Part model, mm, in its own coordinate system. A direction names the side the tool comes from. Give positions to 0.01 mm unless a question says otherwise; leave off trailing zeros. Write each loop counter-clockwise with the first axis right and the second up, starting at its lowest first coordinate (ties: lowest second). Pieces come first, ordered by that corner, then holes. Notation, with made-up numbers: M -2,-7.75 L 57,-7.75 A13 cw 57,9.25 Z; hole C 17,86 d10. An arc over 180 degrees is marked long. Use a Markdown table: item, result. Add a question column.
from build123d import *

# Parameters (mm, degrees)
SKETCH1_W                = 17.4625
SKETCH1_H                = 11.1125
BOSS_EXTRUDE1_DEPTH      = 11.1125
SKETCH2_W                = 20.6375
SKETCH2_H                = 14.2875
BOSS_EXTRUDE2_DEPTH      = 3.048
CHAMFER1_SIZE            = 1.5875
SKETCH3_W                = 15.875
SKETCH3_H                = 9.525
CUT_EXTRUDE1_DEPTH       = 3.175
BOSS_EXTRUDE3_DEPTH      = 4.7498
BOSS_EXTRUDE3_DEPTH_BACK = 4.7498
SKETCH5_W                = 0.762
SKETCH5_H                = 6.0325
BOSS_EXTRUDE4_DEPTH      = 7.62
FILLET1_R                = 1.27


with BuildPart() as part:
    # Sketch1 → Boss-Extrude1 (new body)
    with BuildSketch(Plane(origin=(0, 0, 0), x_dir=(1, 0, 0), z_dir=(0, 1, 0))):
        with Locations((8.73125, 5.55625)):
            Rectangle(SKETCH1_W, SKETCH1_H)
    extrude(amount=BOSS_EXTRUDE1_DEPTH)

    # Sketch2 → Boss-Extrude2 (add)
    with BuildSketch(Plane(origin=(0, 11.1125, 0), x_dir=(1, 0, 0), z_dir=(0, 1, 0))):
        with Locations((8.73125, 5.55625)):
            Rectangle(SKETCH2_W, SKETCH2_H)
    extrude(amount=BOSS_EXTRUDE2_DEPTH)

    # Chamfer1
    chamfer1_edges = [part.edges().sort_by_distance(p)[0] for p in [
        (-1.5875, 14.1605, -5.55625),
        (8.73125, 14.1605, 1.5875),
        (19.05, 14.1605, -5.55625),
        (8.73125, 14.1605, -12.7),
    ]]
    chamfer(chamfer1_edges, length=CHAMFER1_SIZE)

    # Sketch3 → Cut-Extrude1 (cut)
    with BuildSketch(Plane(origin=(0, 14.1605, 0), x_dir=(1, 0, 0), z_dir=(0, 1, 0))):
        with Locations((8.73125, 5.55625)):
            Rectangle(SKETCH3_W, SKETCH3_H)
    extrude(amount=-CUT_EXTRUDE1_DEPTH, mode=Mode.SUBTRACT)

    # Sketch4 → Boss-Extrude3 (add, two sides: drawn at the far end of the back side and taken through both)
    with BuildSketch(Plane.XY.offset(-5.55625).offset(-BOSS_EXTRUDE3_DEPTH_BACK)):
        with BuildLine():
            Line((1.190625, 10.9855), (16.271875, 10.9855))
            Line((16.271875, 10.9855), (16.271875, 14.1605))
            add(Edge.make_bspline(
                [(16.271875, 14.1605), (16.153461698, 15.632290366), (15.692407357, 17.033048026)],
                knots=[0, 0, 0, 1, 1, 1], degree=2))
            ThreePointArc((15.692407357, 17.033048026), (8.639200608, 14.598783188), (1.190625, 14.1605))
            Line((1.190625, 14.1605), (1.190625, 10.9855))
        make_face()
    extrude(amount=BOSS_EXTRUDE3_DEPTH + BOSS_EXTRUDE3_DEPTH_BACK)

    # Sketch5 → Boss-Extrude4 (add)
    with BuildSketch(Plane.XZ):
        with Locations((2.413, -5.55625)):
            Rectangle(SKETCH5_W, SKETCH5_H)
        with Locations((9.525, -5.55625)):
            Rectangle(SKETCH5_W, SKETCH5_H)
    extrude(amount=BOSS_EXTRUDE4_DEPTH)

    # Fillet1
    fillet1_edges = [part.edges().sort_by_distance(p)[0] for p in [
        (2.413, -7.62, -8.5725),
        (2.413, -7.62, -2.54),
        (9.525, -7.62, -8.5725),
        (9.525, -7.62, -2.54),
    ]]
    fillet(fillet1_edges, radius=FILLET1_R)


solid = part.part
1. Mould opens along Z. For faces 5 (the flat face through (-1.588, 12, -5)), 6 (the flat face through (8.59, 13.38, 0.78)), 7 (the flat face through (1, 10.986, -6)) say: released by +Z, released by -Z, zero draft, split by the parting line, or undercut.
2. Tool access for faces 1 (the flat face through (9.906, -4, -6)), 2 (the flat face through (0.794, 13, -5)), 3 (the flat face through (2.794, -4, -6)), 4 (the flat face through (2.032, -4, -6)): list every direction of +Z, -Z, +X, -X, +Y, -Y with a clear straight run to the whole face (end or side of a thin tool).
3. Cut at D-D (y = 8.75). Write the cut outline in (x, z), then the cut area to 3 significant figures.
4. Drill centre lines: probe 1 along X at (y, z) = (11.75, -3.5); probe 2 along X at (y, z) = (-2.5, -7.25); probe 3 along Z at (x, y) = (9.25, 1.75). Where is each one in solid material? Low to high. Write a range as [from, to].
5. Flat gauge pins, fed straight in: pin 1 (1 mm diameter, centred on x = 4.5, z = -1.5, fed in from +Y); pin 2 (3.5 mm diameter, centred on x = 13, y = 6.5, fed in from +Z); pin 3 (4 mm diameter, centred on x = 12.5, z = -5.5, fed in from -Y). Where does each tip first touch, or does it go through?
6. Cut at B-B (y = -1.5). Write the cut outline in (x, z).
7. Cut at A-A (y = 11.75). Write the cut outline in (x, z), then the cut area to 3 significant figures.
A:
| question | item | result |
|---|---|---|
| 1 | face 5 | zero draft |
| 1 | face 6 | released by +Z |
| 1 | face 7 | undercut |
| 2 | face 1 | +Z, -Z, +X, -Y |
| 2 | face 2 | +Y |
| 2 | face 3 | +Z, -Z, -Y |
| 2 | face 4 | +Z, -Z, -X, -Y |
| 3 | outline | M 0,-11.11 L 17.46,-11.11 L 17.46,0 L 0,0 Z |
| 3 | area | 194 mm² |
| 4 | probe 1 | x = [-1.59, 0.79], [1.19, 16.27], [16.67, 19.05] |
| 4 | probe 2 | x = [2.03, 2.79], [9.14, 9.91] |
| 4 | probe 3 | z = [-11.11, 0] |
| 5 | pin 1 | stops at y = 14.13 |
| 5 | pin 2 | stops at z = 0 |
| 5 | pin 3 | stops at y = 0 |
| 6 | outline | M 2.03,-8.57 L 2.79,-8.57 L 2.79,-2.54 L 2.03,-2.54 Z; M 9.14,-8.57 L 9.91,-8.57 L 9.91,-2.54 L 9.14,-2.54 Z |
| 7 | outline | M -1.59,-12.7 L 19.05,-12.7 L 19.05,1.59 L -1.59,1.59 Z; M 1.19,-10.31 L 16.27,-10.31 L 16.27,-0.81 L 1.19,-0.81 Z; hole M 0.79,-10.32 L 16.67,-10.32 L 16.67,-0.79 L 0.79,-0.79 Z |
| 7 | area | 287 mm² |
